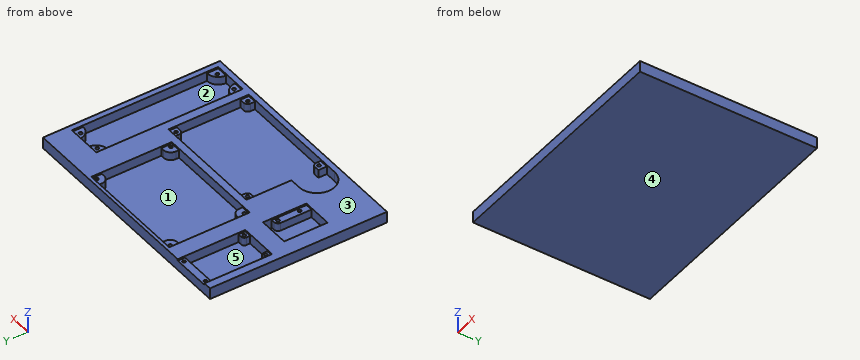
Autodesk Fusion 360 part; units mm, degrees
sketch "Sketch1" plane through (0, 0, 0) normal (0, 0, 1) x (1, 0, 0)
  line L0 (-75, 55) -> (75, 55)
  line L1 (75, 55) -> (75, -55)
  line L2 (75, -55) -> (-75, -55)
  line L3 (-75, -55) -> (-75, 55)
  line L4 (75, -55) -> (-75, 55) construction
  dimension "d1" = 150
  dimension "d2" = 110
extrude "Extrude1" add sketch "Sketch1" along normal blind 1
sketch "Sketch2" plane through (0, 0, 1) normal (0, 0, 1) x (-1, 0, 0)
  line L0 (75, 55) -> (-75, 55)
  line L1 (-75, 55) -> (-75, -55)
  line L2 (-75, -55) -> (75, -55)
  line L3 (75, -55) -> (75, 55)
  line L4 (35.5, -53) -> (-34.5, -53)
  line L5 (-34.5, -53) -> (-34.5, -3)
  line L6 (-34.5, -3) -> (35.5, -3)
  line L7 (35.5, -3) -> (35.5, -53)
  line L8 (26, 1.5) -> (-44, 1.5)
  line L9 (-44, 1.5) -> (-44, 51.5)
  line L10 (-44, 51.5) -> (26, 51.5)
  line L11 (26, 51.5) -> (26, 1.5)
  line L12 (-49.5, -39.5) -> (-71.5, -39.5)
  line L13 (-71.5, -39.5) -> (-71.5, 51.5)
  line L14 (-71.5, 51.5) -> (-49.5, 51.5)
  line L15 (-49.5, 51.5) -> (-49.5, -39.5)
  line L16 (65, -2) -> (46, -2)
  line L17 (46, -2) -> (46, 25)
  line L18 (46, 25) -> (65, 25)
  line L19 (65, 25) -> (65, -2)
  arc A0 (33, 29.5) -> (33, 51.5) centre (33, 40.5) ccw
  line L20 (33, 29.5) -> (26, 29.5)
  line L21 (33, 51.5) -> (26, 51.5)
  line L22 (70, -55) -> (46, -55)
  line L23 (46, -55) -> (46, -13)
  line L24 (46, -13) -> (70, -13)
  line L25 (70, -13) -> (70, -55)
  point P0 (26, 40.5)
  point P1 (33, 40.5)
  dimension "d5" = 70
  dimension "d6" = 50
  dimension "d7" = 70
  dimension "d8" = 50
  dimension "d9" = 22
  dimension "d10" = 91
  dimension "d11" = 19
  dimension "d12" = 27
  dimension "d13" = 3.5
  dimension "d14" = 3.5
  dimension "d15" = 3.5
  dimension "d16" = 2
  dimension "d18" = 10
  dimension "d20" = 20
  dimension "d21" = 5.5
  dimension "d22" = 30
  dimension "d23" = 15
  dimension "d37" = 11
  dimension "d38" = 7
  dimension "d39" = 11
  dimension "d47" = 24
  dimension "d48" = 42
  dimension "d49" = 5
extrude "Extrude2" add sketch "Sketch2" along normal blind 6 contours L0 L1 L2 L3 L23 L24 L25
sketch "Sketch3" plane through (0, 0, 1) normal (0, 0, 1) x (-1, 0, 0)
  line L0 (-71.5, -39.5) -> (-71.5, 51.5)
  line L1 (-71.5, 51.5) -> (-49.5, 51.5)
  line L2 (-49.5, 51.5) -> (-49.5, -39.5)
  line L3 (-49.5, -39.5) -> (-71.5, -39.5)
  circle A0 centre (-53, -36.5) radius 1
  line L4 (-68, 48.5) -> (-53, -36.5) construction
  line L5 (-71.5, -39.5) -> (-49.5, 51.5) construction
  circle A1 centre (-68, -36.5) radius 1
  circle A2 centre (-53, 48.5) radius 1
  circle A3 centre (-68, 48.5) radius 1
  arc A4 (-64.5, -39.5) -> (-71.5, -32.5) centre (-71.5, -39.5) ccw
  arc A5 (-49.5, -32.5) -> (-56.5, -39.5) centre (-49.5, -39.5) ccw
  arc A6 (-71.5, 44.5) -> (-64.5, 51.5) centre (-71.5, 51.5) ccw
  arc A7 (-56.5, 51.5) -> (-49.5, 44.5) centre (-49.5, 51.5) ccw
  dimension "d24" = 2
  dimension "d27" = -15
  dimension "d28" = 85
  dimension "d29" = 7
  dimension "d30" = 7
  dimension "d31" = 7
  dimension "d32" = 7
sketch "Sketch4" plane through (0, 0, 1) normal (0, 0, 1) x (-1, 0, 0)
  line L0 (46, 25) -> (46, -2)
  line L1 (46, -2) -> (65, -2)
  line L2 (65, -2) -> (65, 25)
  line L3 (65, 25) -> (46, 25)
  circle A0 centre (48, 5.9) radius 1
  circle A1 centre (48, 19.4) radius 1
  line L4 (46, -2) -> (46, 25)
  line L5 (46, 25) -> (65, 25)
  arc A2 (48, 3.4) -> (50.5, 5.9) centre (48, 5.9) ccw
  line L6 (48, 3.4) -> (46, 3.4)
  line L7 (50.5, 5.9) -> (50.5, 25)
  dimension "d40" = 2
  dimension "d41" = 2
  dimension "d42" = 13.5
  dimension "d43" = 2
  dimension "d44" = 5.6
  dimension "d45" = 7.9
  dimension "d46" = 2.5
sketch "Sketch5" plane through (0, 0, 1) normal (0, 0, 1) x (-1, 0, 0)
  circle A0 centre (67.7, -52.75) radius 1
  circle A1 centre (48.3, -52.75) radius 1
  circle A2 centre (67.7, -15.25) radius 1
  circle A3 centre (48.3, -15.25) radius 1
  line L0 (67.7, -52.75) -> (48.3, -15.25) construction
  line L1 (46, -13) -> (46, -55) construction
  line L2 (46, -55) -> (70, -55) construction
  line L3 (70, -55) -> (70, -13) construction
  line L4 (70, -13) -> (46, -13) construction
  line L5 (46, -55) -> (70, -13) construction
  line L6 (70, -50.5) -> (46, -50.5)
  line L7 (70, -55) -> (46, -55)
  arc A4 (48.3, -17.25) -> (50.3, -15.25) centre (48.3, -15.25) ccw
  arc A5 (65.7, -15.25) -> (67.7, -17.25) centre (67.7, -15.25) ccw
  line L8 (67.7, -17.25) -> (70, -17.25)
  line L9 (65.7, -15.25) -> (65.7, -13)
  line L10 (50.3, -15.25) -> (50.3, -13)
  line L11 (48.3, -17.25) -> (46, -17.25)
  line L12 (70, -55) -> (70, -50.5)
  line L13 (46, -50.5) -> (46, -55)
  line L14 (50.3, -13) -> (46, -13)
  line L15 (46, -17.25) -> (46, -13)
  line L16 (70, -17.25) -> (70, -13)
  line L17 (70, -13) -> (65.7, -13)
  dimension "d50" = 2
  dimension "d53" = -19.4
  dimension "d54" = 37.5
  dimension "d55" = 2.25
  dimension "d56" = 2.25
  dimension "d57" = 2
  dimension "d58" = 2
sketch "Sketch6" plane through (0, 0, 1) normal (0, 0, 1) x (1, 0, 0)
  line L0 (-35.5, 53) -> (34.5, 53)
  line L1 (-35.5, 3) -> (-35.5, 53)
  line L2 (34.5, 53) -> (34.5, 3)
  line L3 (34.5, 3) -> (-35.5, 3)
  circle A0 centre (-33.5, 5) radius 1
  line L4 (-33.5, 51) -> (32.5, 5) construction
  line L5 (34.5, 53) -> (-35.5, 3) construction
  circle A1 centre (32.5, 5) radius 1
  circle A2 centre (-33.5, 51) radius 1
  circle A3 centre (32.5, 51) radius 1
  arc A4 (-33.5, 46.5) -> (-29, 51) centre (-33.5, 51) ccw
  line L6 (-29, 51) -> (-29, 53)
  line L7 (-33.5, 46.5) -> (-35.5, 46.5)
  line L8 (28, 5) -> (28, 3)
  arc A5 (32.5, 9.5) -> (28, 5) centre (32.5, 5) ccw
  line L9 (32.5, 9.5) -> (34.5, 9.5)
  arc A6 (28, 51) -> (32.5, 46.5) centre (32.5, 51) ccw
  line L10 (32.5, 46.5) -> (34.5, 46.5)
  line L11 (28, 51) -> (28, 53)
  arc A7 (-29, 5) -> (-33.5, 9.5) centre (-33.5, 5) ccw
  line L12 (-33.5, 9.5) -> (-35.5, 9.5)
  line L13 (-29, 5) -> (-29, 3)
  point P0 (-0.5, 28)
  dimension "d59" = 2
  dimension "d62" = 66
  dimension "d63" = 46
  dimension "d64" = 4.5
  dimension "d66" = 360
  dimension "d67" = 4.5
sketch "Sketch7" plane through (0, 0, 1) normal (0, 0, 1) x (-1, 0, 0)
  arc A0 (33, 29.5) -> (33, 51.5) centre (33, 40.5) ccw
  circle A1 centre (-41, 4.25) radius 1
  circle A2 centre (23, 4.25) radius 1
  circle A3 centre (-41, 48.75) radius 1
  circle A4 centre (23, 48.75) radius 1
  line L0 (26, 29.5) -> (26, 1.5) construction
  line L1 (26, 1.5) -> (-44, 1.5) construction
  line L2 (-44, 1.5) -> (-44, 51.5) construction
  line L3 (-44, 51.5) -> (33, 51.5) construction
  line L4 (33, 29.5) -> (26, 29.5) construction
  arc A5 (33, 29.5) -> (33, 51.5) centre (33, 40.5) ccw construction
  line L5 (26, 1.5) -> (-44, 51.5) construction
  line L6 (-41, 4.25) -> (23, 48.75) construction
  arc A6 (23, 6.75) -> (20.5, 4.25) centre (23, 4.25) ccw
  line L7 (20.5, 4.25) -> (20.5, 1.5)
  line L8 (23, 6.75) -> (26, 6.75)
  line L9 (26, 6.75) -> (26, 1.5)
  line L10 (26, 1.5) -> (20.5, 1.5)
  line L11 (-44, 51.5) -> (-38.5, 51.5)
  line L12 (-44, 46.25) -> (-44, 51.5)
  circle A7 centre (-41, 48.75) radius 1
  line L13 (-38.5, 48.75) -> (-38.5, 51.5)
  arc A8 (-41, 46.25) -> (-38.5, 48.75) centre (-41, 48.75) ccw
  line L14 (-41, 46.25) -> (-44, 46.25)
  arc A9 (-38.5, 4.25) -> (-41, 6.75) centre (-41, 4.25) ccw
  line L15 (-41, 4.25) -> (-38.5, 4.25) construction
  line L16 (-41, 4.25) -> (-41, 6.75) construction
  line L17 (-41, 6.75) -> (-44, 6.75)
  line L18 (-38.5, 4.25) -> (-38.5, 1.5)
  line L19 (-38.5, 1.5) -> (-44, 1.5)
  line L20 (-44, 1.5) -> (-44, 6.75)
  line L21 (26, 51.5) -> (26, 46.25)
  line L22 (20.5, 51.5) -> (26, 51.5)
  arc A10 (20.5, 48.75) -> (23, 46.25) centre (23, 48.75) ccw
  line L23 (23, 46.25) -> (26, 46.25)
  line L24 (20.5, 48.75) -> (20.5, 51.5)
  circle A11 centre (23, 48.75) radius 1
  point P0 (-9, 26.5)
  dimension "d77" = 2
  dimension "d80" = 64
  dimension "d81" = 44.5
  dimension "d82" = 2.5
  dimension "d84" = 360
  dimension "d85" = 2.5
  dimension "d86" = 90
extrude "Extrude3" add sketch "Sketch5" sketch "Sketch6" sketch "Sketch3" sketch "Sketch7" sketch "Sketch4" along normal blind 5 of sketch 2 contours L0 L1 A4 L6 L7 | L0 L2 A6 L10 L11 | L1 L3 A7 L12 L13 | L2 L3 L8 A5 L9 of sketch 3 contours L0 L3 A4 | L0 L1 A6 | L2 L3 A5 | L1 L2 A7 of sketch 4 of sketch 5 contours L0 L3 L4 L5 A2 L6 L7
equation "d15 = d14"
equation "d38 = 18 mm - 11 mm"
equation "d56 = d55"
For this review, take the finished solid that the model builds, in its own axes (mm). Face numbers are marked on the shaded views. A direction names the side the tool comes from. Round coordinates to 2 decimals unless told otherwise and drop trailing zeros. Loops run counter-clockwise (first coordinate to the right, second up) from the corner with the lowest first, then second, coordinate; pieces in that order, holes last. Notation, with made-up numbers: (4, -24) - (18, -24) arc R11 ccw to (18, -19) - close; hole circle Ø11 at (-31, 20.25). An arc over 180 degrees is marked (long way). Answer as CSV lines item,"result".
(1) Tool access review of the marked faces 4 and 5: name each direction out of +Z, -Z, +X, -X, +Y, -Y from which nothing blocks a thin tool from reaching the whole face with its end or side.
Checked values:
face 4,"-Z, +X, -X, +Y, -Y"
face 5,"+Z"
(2) Consider section D-D on y = -13.5. Give the boundary of the cut face in (x, z).
Checked values:
outline,"(-75, 0) - (75, 0) - (75, 7) - (71.5, 7) - (71.5, 1) - (49.5, 1) - (49.5, 7) - (44, 7) - (44, 1) - (-26, 1) - (-26, 7) - (-46, 7) - (-46, 6) - (-50.5, 6) - (-50.5, 1) - (-65, 1) - (-65, 7) - (-75, 7) - close"
(3) Mouldability with a two-part tool opening along Y and no side actions: class the marked faces 1, 2 and 3 as +Y half, -Y half, draft (parallel to the pull), parting line (faces both ways), or undercut.
Checked values:
face 1,"undercut"
face 2,"undercut"
face 3,"draft"
(4) Consider section A-A on y = -40.5. Give the boundary of the cut face in (x, z), then the cut area to 3 significant figures.
Checked values:
outline,"(-75, 0) - (75, 0) - (75, 7) - (71.5, 7) - (71.5, 1) - (49.5, 1) - (49.5, 7) - (44, 7) - (44, 1) - (-44, 1) - (-44, 7) - (-75, 7) - close"
area,"390 mm2"
(5) Consider section C-C on z = 4. Give the number of separate pieces and of enclosed holes in the cut face, then the cut area to 3 significant figures.
Checked values:
separate pieces,"1"
enclosed holes,"23"
area,"6,230 mm2"
(6) Wall thickness on line 1 (X direction, y = 46, z = 6.75); line 2 (X direction, y = 29, z = 2.25); line 3 (Y direction, x = 41, z = 3.5): over which ranges is each line inside the solid? List them lowest first.
Checked values:
line 1,"x = -75 to -70, -46 to -35.5, 34.5 to 75"
line 2,"x = -75 to -70, -46 to -35.5, 34.5 to 49.5, 71.5 to 75"
line 3,"y = -55 to -49.75, -47.75 to -46.25, -6.75 to -5.25, -3.25 to 55"
(7) Consider section B-B on x = 14. Give the boundary of the cut face in (y, z), then the cut area to 3 significant figures.
Checked values:
outline,"(-55, 0) - (55, 0) - (55, 7) - (53, 7) - (53, 1) - (3, 1) - (3, 7) - (-1.5, 7) - (-1.5, 1) - (-51.5, 1) - (-51.5, 7) - (-55, 7) - close"
area,"170 mm2"
(8) Insertion check: P1, Ø1.3, axis at x = -53, y = 52.5, coming from the +Z side; P2, Ø1.6, axis at x = -33.5, y = 5, coming from the +Z side. Each pin has a flat end and moves straight along its axis. Give the tip position at first contact, or say it passes through.
Checked values:
P1,"stops at z = 6"
P2,"stops at z = 1"
